Build history of the part. All positions in model axes, mm. A direction names the side the tool comes from. Round coordinates to 2 decimals unless told otherwise and drop trailing zeros. Write each loop counter-clockwise with the first axis right and the second up, starting at its lowest first coordinate (ties: lowest second). Pieces come first, ordered by that corner, then holes.
1) Saw through at A-A (y = 2). Write the cut outline in (x, z).
2) Pull direction X, two halves, no side cores. Call faces 3 (the flat face through (0, 13, 1)), 4 (the flat face through (11, 0, 1)), 5 (the flat face through (11, 26, 1)), 6 (the cylindrical face through (22.699, 0.285, 1.014)): +X half, -X half, draft (parallel to the pull), parting line (faces both ways), or undercut.
3) Which spindle directions (+Z, -Z, +X, -X, +Y, -Y) get a long thin tool onto all of the face, cutting with end or side? Do faces 1 (the flat face through (1, 13, 1)), 2 (the cylindrical face through (0.285, 0.301, 1.014)). Say none if no direction does.
4) Wall check: probe 1 along Y at (x, z) = (13, 0.3); probe 2 along X at (y, z) = (3, 1.6). Give the ranges that are in metal, low to high.
5) Saw through at B-B (x = 19.75). Write the cut outline in (y, z).
6) Saw through at C-C (z = 1.2). Write the cut outline in (x, y).
7) Flat gauge pin, fed straight in: pin 1 (4 mm diameter, centred on x = 8.5, y = 4, fed in from +Z). Where does the tip first touch, or does it go through?
from build123d import *

# Parameters (mm, degrees)
F0_W     = 23
F0_H     = 27
F1_DEPTH = 2
F2_W     = 21
F2_H     = 25
F3_DEPTH = 2.001
F4_R     = 1


with BuildPart() as f1:
    # F0 (on Top) → F1 (new body)
    with BuildSketch(Plane.XY):
        with Locations((11.5, 13.5)):
            Rectangle(F0_W, F0_H)
    extrude(amount=F1_DEPTH)

    # F2 (on face) → F3 (cut, through all)
    with BuildSketch(Plane.XY.offset(2)):
        with Locations((11.5, 13.5)):
            Rectangle(F2_W, F2_H)
    extrude(amount=-F3_DEPTH, mode=Mode.SUBTRACT)

    # F4
    f4_edges = [f1.edges().sort_by_distance(p)[0] for p in [
        (23, 0, 1),
        (23, 27, 1),
        (0, 0, 1),
        (0, 27, 1),
    ]]
    fillet(f4_edges, radius=F4_R)


solid = f1.part
Evaluation:
1. outline: (0, 0) - (1, 0) - (1, 2) - (0, 2) - close; (22, 0) - (23, 0) - (23, 2) - (22, 2) - close
2. face 3: -X half
2. face 4: draft
2. face 5: undercut
2. face 6: +X half
3. face 1: +Z, -Z
3. face 2: +Z, -Z, -X, -Y
4. probe 1: y = 0 to 1, 26 to 27
4. probe 2: x = 0 to 1, 22 to 23
5. outline: (0, 0) - (1, 0) - (1, 2) - (0, 2) - close; (26, 0) - (27, 0) - (27, 2) - (26, 2) - close
6. outline: (0, 1) arc R1 ccw to (1, 0) - (22, 0) arc R1 ccw to (23, 1) - (23, 26) arc R1 ccw to (22, 27) - (1, 27) arc R1 ccw to (0, 26) - close; hole (1, 1) - (22, 1) - (22, 26) - (1, 26) - close
7. pin 1: passes through
